For this review, take the finished solid that the model builds, in its own axes (mm). Face numbers are marked on the shaded views. A direction names the side the tool comes from. Give positions to 0.01 mm unless a question says otherwise; leave off trailing zeros. Order: outer loops, then holes, each group sorted by start corner. A loop starts at its lowest first (then second) coordinate and runs counter-clockwise, first axis right, second up.
Item 1: Machinability: for the marked faces 1, 2 and 3, which of the approach directions +Z, -Z, +X, -X, +Y, -Y give a long, thin tool a straight path to every point of the face, cutting with its end or side? Answer none if there is none.
Item 2: The part is to be moulded in two halves that separate along Y. For the marked faces 4, 5 and 6, say which applies: released by +Y, released by -Y, zero draft, split by the parting line, or undercut.
Item 3: Consider section D-D (y = 6.5). Give the boundary of the cut face in (x, z).
Item 4: Consider section B-B (y = 2.75). Give the boundary of the cut face in (x, z), plus the area to 3 significant figures.
Item 5: For probe 1 along Y at (x, z) = (10, 0.7); probe 2 along Y at (x, z) = (-14, 9); probe 3 along X at (y, z) = (2.65, 10), list the stretches that pass through material, from the lowest coordinate up.
Item 6: For P1, Ø6, axis at y = 10, z = 4, coming from the -X side; P2, Ø4.5, axis at x = 9.5, z = 10, coming from the +Y side; P3, Ø3.5, axis at x = -14, y = 10, coming from the -Z side; P4, Ø3, axis at y = 9, z = 7, coming from the +X side, all flat-tipped, find the tip position at first contact; note any pin that passes through.
Item 7: Consider section C-C (x = 9). Give the boundary of the cut face in (y, z), plus the area to 3 significant figures.
Item 8: Consider section A-A (z = 10). Give the boundary of the cut face in (x, y), plus the area to 3 significant figures.
```python
from build123d import *

# Parameters (mm, degrees)
ESQUISSE1_R             = 2.1
BOSS_EXTRU_1_DEPTH      = 5
ESQUISSE2_W             = 12
ESQUISSE2_H             = 11
ESQUISSE2_W_2           = 20
ESQUISSE2_H_2           = 3
BOSS_EXTRU_2_DEPTH      = 10
ESQUISSE3_R             = 2.8
ENL_V_MAT_EXTRU_1_DEPTH = 9.1
ESQUISSE4_R             = 2.1
ENL_V_MAT_EXTRU_2_DEPTH = 9.1
CONG_2_R                = 2


with BuildPart() as part:
    # Esquisse1 → Boss.-Extru.1 (new body)
    with BuildSketch(Plane(origin=(0, 0, 0), x_dir=(1, 0, 0), z_dir=(0, 1, 0))):
        Polygon((20, 0), (20, -15), (-20, -15), (-20, -4), (0, 0), align=None)
        with Locations(Location((5, -10, 0), (0, 0, 270))):
            Circle(ESQUISSE1_R, mode=Mode.SUBTRACT)
    extrude(amount=BOSS_EXTRU_1_DEPTH)

    # Esquisse2 → Boss.-Extru.2 (add)
    with BuildSketch(Plane(origin=(0, 5, 0), x_dir=(1, 0, 0), z_dir=(0, 1, 0))):
        with Locations((-14, -9.5)):
            Rectangle(ESQUISSE2_W, ESQUISSE2_H)
        with Locations((10, -1.5)):
            Rectangle(ESQUISSE2_W_2, ESQUISSE2_H_2)
        Polygon((-8, -4), (-8, -1.6), (-20, -4), align=None)
    extrude(amount=BOSS_EXTRU_2_DEPTH)

    # Esquisse3 → Enl_v. mat.-Extru.1 (cut)
    with BuildSketch(Plane.XY.offset(15)):
        with Locations((-14, 10)):
            Circle(ESQUISSE3_R)
    extrude(amount=-ENL_V_MAT_EXTRU_1_DEPTH, mode=Mode.SUBTRACT)

    # Esquisse4 → Enl_v. mat.-Extru.2 (cut)
    with BuildSketch(Plane.XY.offset(3)):
        with Locations((10, 10)):
            Circle(ESQUISSE4_R)
    extrude(amount=-ENL_V_MAT_EXTRU_2_DEPTH, mode=Mode.SUBTRACT)

    # Cong_2
    cong_2_edges = [part.edges().sort_by_distance(p)[0] for p in [
        (0, 10, 3),
        (20, 10, 3),
        (-8, 10, 1.6),
        (-20, 7.5, 4),
    ]]
    fillet(cong_2_edges, radius=CONG_2_R)


solid = part.part
```
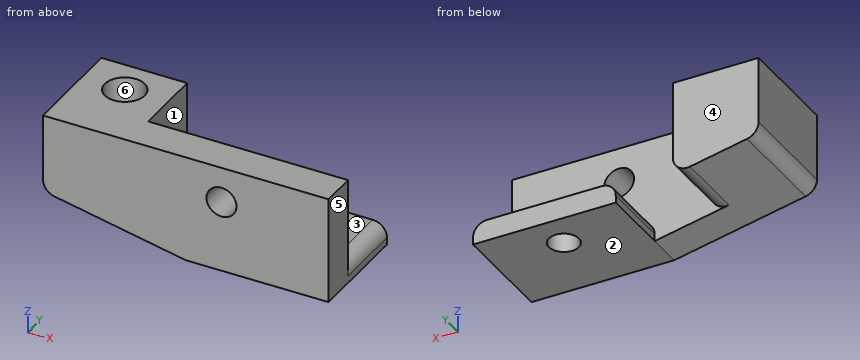
Resolved:
1. face 1: +Z, -Z, +X, +Y
1. face 2: -Z, +X, -X, +Y, -Y
1. face 3: +Z, +X, +Y
2. face 4: released by +Y
2. face 5: zero draft
2. face 6: undercut
3. outline: (-20, 5.64) arc R2 ccw to (-18.39, 3.68) - (-10.39, 2.08) arc R2 ccw to (-8, 4.04) - (-8, 15) - (-20, 15) - close; (0, 0) - (20, 0) - (20, 1) arc R2 ccw to (18, 3) - (2, 3) arc R2 ccw to (0, 1) - close
4. outline: (-20, 5.64) arc R2 ccw to (-18.39, 3.68) - (0, 0) - (20, 0) - (20, 15) - (-20, 15) - close; hole circle Ø4.2 at (5, 10)
4. area: 546 mm2
5. probe 1: y = 0 to 7.9, 12.1 to 15
5. probe 2: y = 0 to 7.2, 12.8 to 15
5. probe 3: x = -20 to 2.9, 7.1 to 20
6. P1: stops at x = -20
6. P2: stops at y = 5
6. P3: stops at z = 2.45
6. P4: stops at x = -8
7. outline: (0, 0) - (8.15, 0) - (8.15, 3) - (5, 3) - (5, 15) - (0, 15) - close; (11.85, 0) - (15, 0) - (15, 3) - (11.85, 3) - close
7. area: 93.9 mm2
8. outline: (-20, 0) - (2.9, 0) - (2.9, 5) - (-8, 5) - (-8, 15) - (-20, 15) - close; (7.1, 0) - (20, 0) - (20, 5) - (7.1, 5) - close; hole circle Ø5.6 at (-14, 10)
8. area: 274 mm2
